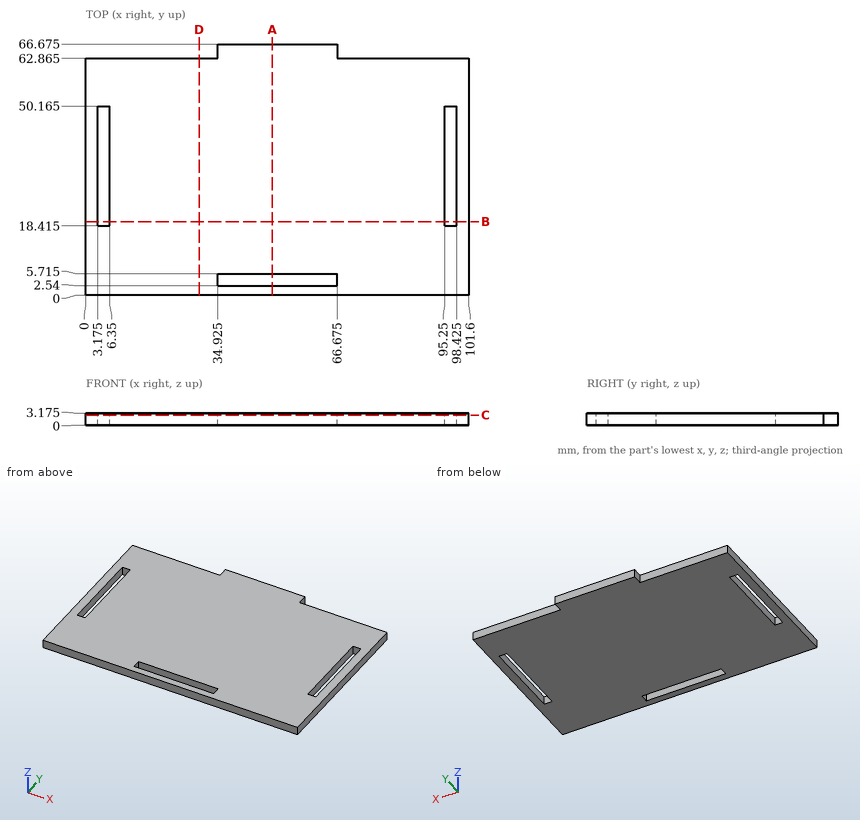
Here's the drawing with two shaded views (mm, measured from the low corner). I have some questions. Coordinates: 2 decimals unless noted, no trailing zeros. Loops run counter-clockwise (first coordinate to the right, second up) from the corner with the lowest first, then second, coordinate; pieces in that order, holes last.
Item 1: Suppose I cut it at D-D (x = 30). Please give me the cut outline in (y, z) (3 decimals).
Answers below:
outline: (0, 0) - (62.865, 0) - (62.865, 3.175) - (0, 3.175) - close
Item 2: I'm going to push flat-ended pins straight in: pin 1 (1.6 mm diameter, centred on y = 64, z = 1.5, fed in from -X) (3 decimals); pin 2 (1.6 mm diameter, centred on x = 11, z = 2, fed in from +Y) (3 decimals); pin 3 (1 mm diameter, centred on y = 64.5, z = 1.5, fed in from +X) (3 decimals). Where does each tip first touch, or does it pass through?
Answers below:
pin 1: stops at x = 34.925
pin 2: stops at y = 62.865
pin 3: stops at x = 66.675
Item 3: Suppose I cut it at B-B (y = 19.5). Please give me the cut outline in (x, z) (3 decimals).
Answers below:
outline: (0, 0) - (3.175, 0) - (3.175, 3.175) - (0, 3.175) - close; (6.35, 0) - (95.25, 0) - (95.25, 3.175) - (6.35, 3.175) - close; (98.425, 0) - (101.6, 0) - (101.6, 3.175) - (98.425, 3.175) - close
Item 4: Suppose I cut it at A-A (x = 49.5). Please give me the cut outline in (y, z) (3 decimals).
Answers below:
outline: (0, 0) - (2.54, 0) - (2.54, 3.175) - (0, 3.175) - close; (5.715, 0) - (66.675, 0) - (66.675, 3.175) - (5.715, 3.175) - close
Item 5: Please list where these lines run through material, in increasing order: L1, parallel to X at y = 34, z = 0.2 (3 decimals); L2, parallel to Y at x = 52, z = 0.9 (3 decimals); L3, parallel to Y at x = 77.5, z = 2.9 (3 decimals).
Answers below:
L1: x = 0 to 3.175, 6.35 to 95.25, 98.425 to 101.6
L2: y = 0 to 2.54, 5.715 to 66.675
L3: y = 0 to 62.865
Item 6: Suppose I cut it at C-C (z = 2.65). Please give me the cut outline in (x, y) (3 decimals).
Answers below:
outline: (0, 0) - (101.6, 0) - (101.6, 62.865) - (66.675, 62.865) - (66.675, 66.675) - (34.925, 66.675) - (34.925, 62.865) - (0, 62.865) - close; hole (3.175, 18.415) - (6.35, 18.415) - (6.35, 50.165) - (3.175, 50.165) - close; hole (34.925, 2.54) - (66.675, 2.54) - (66.675, 5.715) - (34.925, 5.715) - close; hole (95.25, 18.415) - (98.425, 18.415) - (98.425, 50.165) - (95.25, 50.165) - close
